The listing builds one solid part. Answer for the finished solid, in the listing's coordinates (mm). Face numbers are marked on the shaded views. A direction names the side the tool comes from. Round coordinates to 2 decimals unless told otherwise and drop trailing zeros. Order: outer loops, then holes, each group sorted by start corner. A loop starts at its lowest first (then second) coordinate and runs counter-clockwise, first axis right, second up. Notation, with made-up numbers: (76, 48) - (92, 48) arc R25 ccw to (92, 68) - close; hole circle Ø10 at (7.25, 60). An arc over 180 degrees is marked (long way). One line per item, written item: value. Start each with the question number.
1. Section C-C, the plane z = 38.5 is taken. Give the vertices of the cut face in (x, y) (3 decimals), then the cut area to 3 significant figures.
2. Flat-ended cylindrical pins translate along their axes: P1, Ø5, axis at x = -27.5, z = 39, coming from the +Y side; P2, Ø22, axis at x = -47.5, z = 26, coming from the -Y side; P3, Ø5.5, axis at x = -100, z = 19, coming from the -Y side. Find the tip coordinate at first contact, or state that the pin passes through.
3. Straight lines are drawn through the part: line 1 (X direction, y = 22.5, z = 40); line 2 (Y direction, x = -93.5, z = 20.5); line 3 (X direction, y = 86, z = 17). For each, find the intervals that lie inside material, in ascending order.
4. A tool of negligible diameter and unlimited length cuts with its end or side. For the marked faces 1, 2 and 3, from which of +Z, -Z, +X, -X, +Y, -Y can it reach the whole face along a straight path? Write none if from no direction.
5. Section B-B, the plane x = -44 is taken. Give the vertices of the cut face in (y, z), then the cut area to 3 significant figures.
6. Section D-D, the plane z = 17 is taken. Count the separate pieces of the cut face and the enclosed holes in it, then the cut area to 3 significant figures.
7. Section A-A, the plane x = 10 is taken. Give the vertices of the cut face in (y, z), then the cut area to 3 significant figures.
8. For a pull along Y with two mould halves and no side action, classify the marked faces 4, 5, 6 and 7 as released by +Y, released by -Y, zero draft, split by the parting line, or undercut.
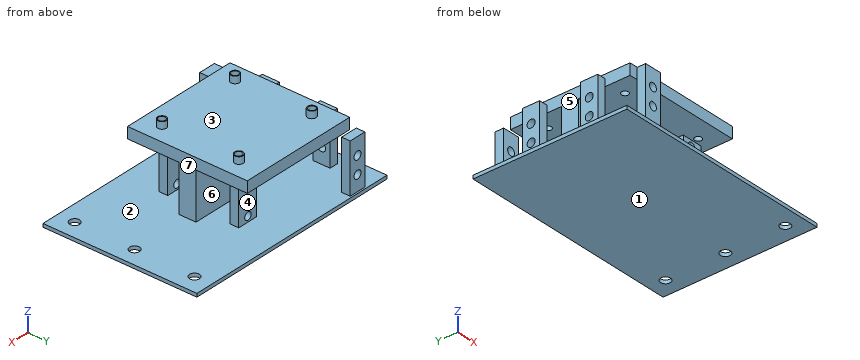
from build123d import *

# Parameters (mm, degrees)
SKETCH058_R                = 2.21
EXTRUDE064_DEPTH           = 10
SKETCH057_R                = 2.21
EXTRUDE063_DEPTH           = 10
SKETCH056_W                = 12
SKETCH056_H                = 26.01178
EXTRUDE062_DEPTH           = 5
SKETCH055_R                = 2.21
EXTRUDE061_DEPTH           = 10
SKETCH054_R                = 2.21
EXTRUDE060_DEPTH           = 10
SKETCH053_W                = 12
SKETCH053_H                = 26.01178
EXTRUDE059_DEPTH           = 5
SKETCH048_R                = 2.34
EXTRUDE050_DEPTH           = 20
SKETCH047_W                = 10
SKETCH047_H                = 30
EXTRUDE049_DEPTH           = 5
EXTRUDE049_PLACEMENT_ANGLE = 90
CUT029_PLACEMENT_ANGLE     = 90
SKETCH040_R                = 2.34
EXTRUDE042_DEPTH           = 20
SKETCH039_W                = 10
SKETCH039_H                = 30
EXTRUDE041_DEPTH           = 5
EXTRUDE041_PLACEMENT_ANGLE = 90
SKETCH038_R                = 2.34
EXTRUDE039_DEPTH           = 20
SKETCH037_W                = 10
SKETCH037_H                = 30
EXTRUDE038_DEPTH           = 5
EXTRUDE038_PLACEMENT_ANGLE = 90
SKETCH046_R                = 2.34
EXTRUDE048_DEPTH           = 20
SKETCH045_W                = 10
SKETCH045_H                = 30
EXTRUDE047_DEPTH           = 5
EXTRUDE047_PLACEMENT_ANGLE = 90
CUT026_PLACEMENT_ANGLE     = 90
SKETCH016_R                = 2.005
EXTRUDE058_DEPTH           = 20
EXTRUDE057_DEPTH           = 20
EXTRUDE056_DEPTH           = 20
EXTRUDE055_DEPTH           = 20
SKETCH015_R                = 2.5
EXTRUDE054_DEPTH           = 8
EXTRUDE053_DEPTH           = 70
EXTRUDE053_PLACEMENT_ANGLE = 90
SKETCH051_R                = 2.9
EXTRUDE052_DEPTH           = 50
SKETCH050_W                = 130
SKETCH050_H                = 90
EXTRUDE051_DEPTH           = 2


with BuildPart() as extrude064:
    # Sketch058 → Extrude064 (new body)
    with BuildSketch(Plane.XZ):
        with Locations((-30.242167, 20.01615)):
            Circle(SKETCH058_R)
    extrude(amount=EXTRUDE064_DEPTH)


with BuildPart() as extrude064_1:
    # Extrude064 placement: moved
    add(extrude064.part.moved(Location((-9.8, 5, -14.82))))


with BuildPart() as extrude063:
    # Sketch057 → Extrude063 (new body)
    with BuildSketch(Plane.XZ):
        with Locations((-30.242167, 20.01615)):
            Circle(SKETCH057_R)
    extrude(amount=EXTRUDE063_DEPTH)


with BuildPart() as extrude063_1:
    # Extrude063 placement: moved
    add(extrude063.part.moved(Location((-9.8, 3, 2.68))))


with BuildPart() as cut035:
    # Sketch056 → Extrude062 (new body)
    with BuildSketch(Plane.XZ):
        with Locations((-39.733391, 13.00589)):
            Rectangle(SKETCH056_W, SKETCH056_H)
    extrude(amount=EXTRUDE062_DEPTH)

    # Cut034: cut Extrude063
    add(extrude063_1.part, mode=Mode.SUBTRACT)

    # Cut035: cut Extrude064
    add(extrude064_1.part, mode=Mode.SUBTRACT)


with BuildPart() as cut035_1:
    # Cut035 placement: moved
    add(cut035.part.moved(Location((0, 68.5, 6))))


with BuildPart() as extrude061:
    # Sketch055 → Extrude061 (new body)
    with BuildSketch(Plane.XZ):
        with Locations((-30.242167, 20.01615)):
            Circle(SKETCH055_R)
    extrude(amount=EXTRUDE061_DEPTH)


with BuildPart() as extrude061_1:
    # Extrude061 placement: moved
    add(extrude061.part.moved(Location((-9.8, 5, -14.82))))


with BuildPart() as extrude060:
    # Sketch054 → Extrude060 (new body)
    with BuildSketch(Plane.XZ):
        with Locations((-30.242167, 20.01615)):
            Circle(SKETCH054_R)
    extrude(amount=EXTRUDE060_DEPTH)


with BuildPart() as extrude060_1:
    # Extrude060 placement: moved
    add(extrude060.part.moved(Location((-9.8, 3, 2.68))))


with BuildPart() as cut033:
    # Sketch053 → Extrude059 (new body)
    with BuildSketch(Plane.XZ):
        with Locations((-39.733391, 13.00589)):
            Rectangle(SKETCH053_W, SKETCH053_H)
    extrude(amount=EXTRUDE059_DEPTH)

    # Cut032: cut Extrude060
    add(extrude060_1.part, mode=Mode.SUBTRACT)

    # Cut033: cut Extrude061
    add(extrude061_1.part, mode=Mode.SUBTRACT)


with BuildPart() as cut033_1:
    # Cut033 placement: moved
    add(cut033.part.moved(Location((0, 27, 6))))


with BuildPart() as tornillos010:
    # Sketch048 (on Face6 of Extrude049) → Extrude050 (new body)
    with BuildSketch(Plane(origin=(-101, -107, 0), x_dir=(0, -1, 0), z_dir=(-1, 0, 0))):
        with Locations((-135.006037, 30)):
            Circle(SKETCH048_R)
        with Locations((-135.008375, 20)):
            Circle(SKETCH048_R)
    extrude(amount=EXTRUDE050_DEPTH)


with BuildPart() as tornillos010_1:
    # Extrude050 placement: moved
    add(tornillos010.part.moved(Location((17, 0, 0))))


with BuildPart() as soporte012:
    # Sketch047 → Extrude049 (new body)
    with BuildSketch(Plane.XZ):
        with Locations((-135, 25)):
            Rectangle(SKETCH047_W, SKETCH047_H)
    extrude(amount=EXTRUDE049_DEPTH)


with BuildPart() as soporte012_1:
    # Extrude049 placement: moved
    add(soporte012.part.moved(Location((-96, -107, 0))).rotate(Axis((-96, -107, 0), (0, 0, -1)), EXTRUDE049_PLACEMENT_ANGLE))

    # Cut029: cut Tornillos010
    add(tornillos010_1.part, mode=Mode.SUBTRACT)


with BuildPart() as soporte012_2:
    # Cut029 placement: moved
    add(soporte012_1.part.moved(Location((-119, -12, -3))).rotate(Axis((-119, -12, -3), (0, 0, -1)), CUT029_PLACEMENT_ANGLE))


with BuildPart() as tornillos007:
    # Sketch040 (on Face6 of Extrude041) → Extrude042 (new body)
    with BuildSketch(Plane(origin=(-101, -107, 0), x_dir=(0, -1, 0), z_dir=(-1, 0, 0))):
        with Locations((-135.006037, 30)):
            Circle(SKETCH040_R)
        with Locations((-135.008375, 20)):
            Circle(SKETCH040_R)
    extrude(amount=EXTRUDE042_DEPTH)


with BuildPart() as tornillos007_1:
    # Extrude042 placement: moved
    add(tornillos007.part.moved(Location((17, 0, 0))))


with BuildPart() as soporte011:
    # Sketch039 → Extrude041 (new body)
    with BuildSketch(Plane.XZ):
        with Locations((-135, 25)):
            Rectangle(SKETCH039_W, SKETCH039_H)
    extrude(amount=EXTRUDE041_DEPTH)


with BuildPart() as soporte011_1:
    # Extrude041 placement: moved
    add(soporte011.part.moved(Location((-96, -107, 0))).rotate(Axis((-96, -107, 0), (0, 0, -1)), EXTRUDE041_PLACEMENT_ANGLE))

    # Cut028: cut Tornillos007
    add(tornillos007_1.part, mode=Mode.SUBTRACT)


with BuildPart() as soporte011_2:
    # Cut028 placement: moved
    add(soporte011_1.part.moved(Location((-2, 34, -3))))


with BuildPart() as tornillos005:
    # Sketch038 (on Face6 of Extrude038) → Extrude039 (new body)
    with BuildSketch(Plane(origin=(-101, -107, 0), x_dir=(0, -1, 0), z_dir=(-1, 0, 0))):
        with Locations((-135.006037, 30)):
            Circle(SKETCH038_R)
        with Locations((-135.008375, 20)):
            Circle(SKETCH038_R)
    extrude(amount=EXTRUDE039_DEPTH)


with BuildPart() as tornillos005_1:
    # Extrude039 placement: moved
    add(tornillos005.part.moved(Location((17, 0, 0))))


with BuildPart() as soporte010:
    # Sketch037 → Extrude038 (new body)
    with BuildSketch(Plane.XZ):
        with Locations((-135, 25)):
            Rectangle(SKETCH037_W, SKETCH037_H)
    extrude(amount=EXTRUDE038_DEPTH)


with BuildPart() as soporte010_1:
    # Extrude038 placement: moved
    add(soporte010.part.moved(Location((-96, -107, 0))).rotate(Axis((-96, -107, 0), (0, 0, -1)), EXTRUDE038_PLACEMENT_ANGLE))

    # Cut027: cut Tornillos005
    add(tornillos005_1.part, mode=Mode.SUBTRACT)


with BuildPart() as soporte010_2:
    # Cut027 placement: moved
    add(soporte010_1.part.moved(Location((-2, 0, -3))))


with BuildPart() as tornillos009:
    # Sketch046 (on Face6 of Extrude047) → Extrude048 (new body)
    with BuildSketch(Plane(origin=(-101, -107, 0), x_dir=(0, -1, 0), z_dir=(-1, 0, 0))):
        with Locations((-135.006037, 30)):
            Circle(SKETCH046_R)
        with Locations((-135.008375, 20)):
            Circle(SKETCH046_R)
    extrude(amount=EXTRUDE048_DEPTH)


with BuildPart() as tornillos009_1:
    # Extrude048 placement: moved
    add(tornillos009.part.moved(Location((17, 0, 0))))


with BuildPart() as soporte009:
    # Sketch045 → Extrude047 (new body)
    with BuildSketch(Plane.XZ):
        with Locations((-135, 25)):
            Rectangle(SKETCH045_W, SKETCH045_H)
    extrude(amount=EXTRUDE047_DEPTH)


with BuildPart() as soporte009_1:
    # Extrude047 placement: moved
    add(soporte009.part.moved(Location((-96, -107, 0))).rotate(Axis((-96, -107, 0), (0, 0, -1)), EXTRUDE047_PLACEMENT_ANGLE))

    # Cut026: cut Tornillos009
    add(tornillos009_1.part, mode=Mode.SUBTRACT)


with BuildPart() as soporte009_2:
    # Cut026 placement: moved
    add(soporte009_1.part.moved(Location((-119, -95, -3))).rotate(Axis((-119, -95, -3), (0, 0, -1)), CUT026_PLACEMENT_ANGLE))


with BuildPart() as tornillo008:
    # Sketch016 (on Face16 of Fusion001) → Extrude058 (new body)
    with BuildSketch(Plane.XY.offset(45.913223)):
        with Locations((-84.962639, 67.504814)):
            Circle(SKETCH016_R)
    extrude(amount=EXTRUDE058_DEPTH)


with BuildPart() as tornillo008_1:
    # Extrude058 placement: moved
    add(tornillo008.part.moved(Location((0, -45, -17))))


with BuildPart() as tornillo007:
    # Sketch016 (on Face16 of Fusion001) → Extrude057 (new body)
    with BuildSketch(Plane.XY.offset(45.913223)):
        with Locations((-84.962639, 67.504814)):
            Circle(SKETCH016_R)
    extrude(amount=EXTRUDE057_DEPTH)


with BuildPart() as tornillo007_1:
    # Extrude057 placement: moved
    add(tornillo007.part.moved(Location((50, -45, -15))))


with BuildPart() as tornillo006:
    # Sketch016 (on Face16 of Fusion001) → Extrude056 (new body)
    with BuildSketch(Plane.XY.offset(45.913223)):
        with Locations((-84.962639, 67.504814)):
            Circle(SKETCH016_R)
    extrude(amount=EXTRUDE056_DEPTH)


with BuildPart() as tornillo006_1:
    # Extrude056 placement: moved
    add(tornillo006.part.moved(Location((0, 0, -15))))


with BuildPart() as tornillo005:
    # Sketch016 (on Face16 of Fusion001) → Extrude055 (new body)
    with BuildSketch(Plane.XY.offset(45.913223)):
        with Locations((-84.962639, 67.504814)):
            Circle(SKETCH016_R)
    extrude(amount=EXTRUDE055_DEPTH)


with BuildPart() as tornillo005_1:
    # Extrude055 placement: moved
    add(tornillo005.part.moved(Location((50.1, 0, -18))))


with BuildPart() as tornillos012:
    # Sketch015 (on Face16 of Fusion) → Extrude054 (new body)
    with BuildSketch(Plane.XY.offset(41.913223)):
        with Locations((-84.986267, 67.433998)):
            Circle(SKETCH015_R)
        with Locations((-85.013062, 22.499535)):
            Circle(SKETCH015_R)
        with Locations((-35.024185, 22.542374)):
            Circle(SKETCH015_R)
        with Locations((-34.910458, 67.59893)):
            Circle(SKETCH015_R)
    extrude(amount=EXTRUDE054_DEPTH)


with BuildPart() as tornillos012_1:
    # Extrude054 placement: moved
    add(tornillos012.part.moved(Location((0, 0, -4))))


with BuildPart() as obj1:
    # Sketch052 → Extrude053 (new body)
    with BuildSketch(Plane.XZ):
        Polygon((-100, 9.995709), (-100, 37.355709), (-130, 37.355709), (-130, 43.915709), (-60, 43.915709), (-60, 37.355709), (-90, 37.355709), (-90, 9.995709), align=None)
    extrude(amount=EXTRUDE053_DEPTH)


with BuildPart() as obj1_1:
    # Extrude053 placement: moved
    add(obj1.part.moved(Location((-25, -49, -2))).rotate(Axis((-25, -49, -2), (0, 0, -1)), EXTRUDE053_PLACEMENT_ANGLE))


with BuildPart() as tornillos011:
    # Sketch051 (on Face6 of Extrude051) → Extrude052 (new body)
    with BuildSketch(Plane.XY.offset(2)):
        with Locations((120, 80.020506)):
            Circle(SKETCH051_R)
        with Locations((120, 45.010253)):
            Circle(SKETCH051_R)
        with Locations((120, 10)):
            Circle(SKETCH051_R)
    extrude(amount=EXTRUDE052_DEPTH)


with BuildPart() as tornillos011_1:
    # Extrude052 placement: moved
    add(tornillos011.part.moved(Location((0, 0, -31))))


with BuildPart() as no:
    # Sketch050 → Extrude051 (new body)
    with BuildSketch(Plane.XY):
        with Locations((65, 45)):
            Rectangle(SKETCH050_W, SKETCH050_H)
    extrude(amount=EXTRUDE051_DEPTH)

    # Cut021: cut Tornillos011
    add(tornillos011_1.part, mode=Mode.SUBTRACT)


with BuildPart() as no_1:
    # Cut021 placement: moved
    add(no.part.moved(Location((-110, 0, 6))))

    # Fusion010: union obj1
    add(obj1_1.part)

    # Fusion011: union Tornillos012
    add(tornillos012_1.part)

    # Cut022: cut Tornillo005
    add(tornillo005_1.part, mode=Mode.SUBTRACT)

    # Cut023: cut Tornillo006
    add(tornillo006_1.part, mode=Mode.SUBTRACT)

    # Cut024: cut Tornillo007
    add(tornillo007_1.part, mode=Mode.SUBTRACT)

    # Cut025: cut Tornillo008
    add(tornillo008_1.part, mode=Mode.SUBTRACT)

    # Fusion012: union Soporte009
    add(soporte009_2.part)

    # Fusion013: union Soporte010
    add(soporte010_2.part)

    # Fusion014: union Soporte011
    add(soporte011_2.part)

    # Fusion015: union Soporte012
    add(soporte012_2.part)

    # Fusion016: union Cut033
    add(cut033_1.part)

    # Fusion017: union Cut035
    add(cut035_1.part)


solid = no_1.part
Answer list:
1. outline: (-95, 11) - (-25, 11) - (-25, 81) - (-95, 81) - close; hole circle Ø4.01 at (-84.963, 22.505); hole circle Ø4.01 at (-84.963, 67.505); hole circle Ø4.01 at (-34.963, 22.505); hole circle Ø4.01 at (-34.863, 67.505)
1. area: 4,850 mm²
2. P1: stops at y = 81
2. P2: stops at y = 11
2. P3: stops at y = 23
3. line 1: x = -95 to -86.97, -82.96 to -36.97, -32.96 to -25
3. line 2: y = 1 to 6, 41 to 51, 84 to 89
3. line 3: x = -96 to -93.33, -88.65 to -86
4. face 1: -Z, +X, -X, +Y, -Y
4. face 2: none
4. face 3: +Z
5. outline: (0, 6) - (90, 6) - (90, 8) - (68.5, 8) - (68.5, 32.01) - (63.5, 32.01) - (63.5, 8) - (51, 8) - (51, 35.36) - (81, 35.36) - (81, 41.92) - (11, 41.92) - (11, 35.36) - (41, 35.36) - (41, 8) - (27, 8) - (27, 32.01) - (22, 32.01) - (22, 8) - (0, 8) - close
5. area: 1,150 mm²
6. separate pieces: 11
6. enclosed holes: 0
6. area: 926 mm²
7. outline: (0, 6) - (7.1, 6) - (7.1, 8) - (0, 8) - close; (12.9, 6) - (42.11, 6) - (42.11, 8) - (12.9, 8) - close; (47.91, 6) - (77.12, 6) - (77.12, 8) - (47.91, 8) - close; (82.92, 6) - (90, 6) - (90, 8) - (82.92, 8) - close
7. area: 145 mm²
8. face 4: released by +Y
8. face 5: undercut
8. face 6: undercut
8. face 7: zero draft
